Could you check a few things on this drawing? It's one solid part, dimensions in mm from its lowest x, y, z. Coordinates: 2 decimals unless noted, no trailing zeros. Order: outer loops, then holes, each group sorted by start corner. A loop starts at its lowest first (then second) coordinate and runs counter-clockwise, first axis right, second up. Notation, with made-up numbers: (57.25, -37) -> (92.25, -37) arc R21 ccw to (92.25, -4) -> close; hole circle Ø9 at (80, -22.75). An arc over 180 degrees is marked (long way). Use a Markdown table: item, result. Add a question column.
1. Suppose I cut it at B-B, the plane x = 63. List the corners of the cut face in (y, z) for me.
2. For pin 1 Ø10 at (x, z) = (33.5, 32.5) entering from -Y; pin 2 Ø2 at (x, z) = (63, 57.5) entering from +Y, each with a flat end and sliding along its axis, tell me the tip position at first contact or that it passes through.
3. Suppose I cut it at A-A, the plane z = 17.5. List the corners of the cut face in (x, y) for me.
4. If I drill on line 1 along X through (y, z) = (0.9, 17.5); line 2 along Z through (x, y) = (64, 0.2); line 3 along X through (y, z) = (1, 18.5), over which ranges is the centre line in solid material (lowest first)? Write a range as from..to.
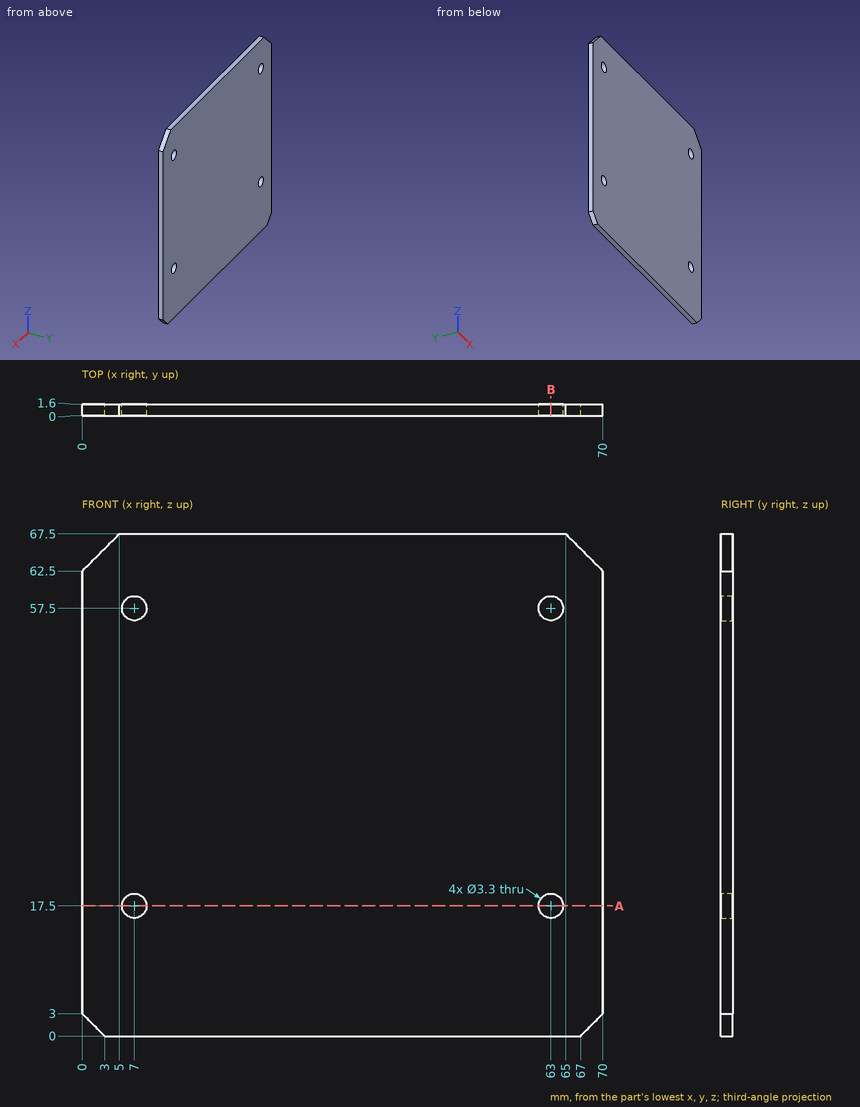
Worked out:
| question | item | result |
|---|---|---|
| 1 | outline | (0, 0) -> (1.6, 0) -> (1.6, 15.85) -> (0, 15.85) -> close; (0, 19.15) -> (1.6, 19.15) -> (1.6, 55.85) -> (0, 55.85) -> close; (0, 59.15) -> (1.6, 59.15) -> (1.6, 67.5) -> (0, 67.5) -> close |
| 2 | pin 1 | stops at y = 0 |
| 2 | pin 2 | passes through |
| 3 | outline | (0, 0) -> (5.35, 0) -> (5.35, 1.6) -> (0, 1.6) -> close; (8.65, 0) -> (61.35, 0) -> (61.35, 1.6) -> (8.65, 1.6) -> close; (64.65, 0) -> (70, 0) -> (70, 1.6) -> (64.65, 1.6) -> close |
| 4 | line 1 | x = 0..5.35, 8.65..61.35, 64.65..70 |
| 4 | line 2 | z = 0..16.19, 18.81..56.19, 58.81..67.5 |
| 4 | line 3 | x = 0..5.69, 8.31..61.69, 64.31..70 |
